from build123d import *

# Parameters (mm, degrees)
SKETCH_1_W          = 1150
SKETCH_1_H          = 15
EXTRUDE_1_DEPTH     = 30
SKETCH_2_R          = 7
CUT_EXTRUDE_1_DEPTH = 1195.521313651


with BuildPart() as part:
    # Эскиз1 → Бобышка-Вытянуть1 (new body)
    with BuildSketch(Plane.XY):
        with Locations((619.050320868, 30.131091658)):
            Rectangle(SKETCH_1_W, SKETCH_1_H)
    extrude(amount=EXTRUDE_1_DEPTH)

    # Эскиз2 → Вырез-Вытянуть1 (cut, through all)
    with BuildSketch(Plane(origin=(0, 37.631091658, 0), x_dir=(1, 0, 0), z_dir=(0, 1, 0))):
        with Locations(Location((144.050320868, -15, 0), (0, 0, 270))):
            Circle(SKETCH_2_R)
        with Locations(Location((614.050320868, -15, 0), (0, 0, 270))):
            Circle(SKETCH_2_R)
        with Locations(Location((1084.050320868, -15, 0), (0, 0, 270))):
            Circle(SKETCH_2_R)
    extrude(amount=-CUT_EXTRUDE_1_DEPTH, mode=Mode.SUBTRACT)


solid = part.part
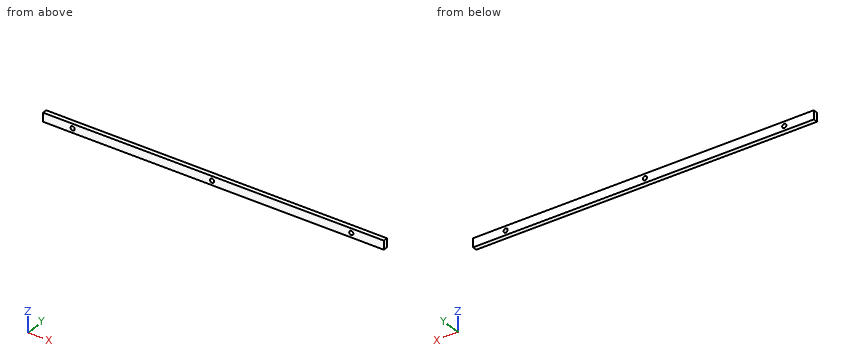
The model under review builds one solid part; all positions refer to its coordinate system, in mm. Give positions to 0.01 mm unless a question says otherwise; leave off trailing zeros. Order: outer loops, then holes, each group sorted by start corner. A loop starts at its lowest first (then second) coordinate and runs counter-clockwise, first axis right, second up. Notation, with made-up numbers: M 89.25,7.5 L 118.25,7.5 A18 cw 118.25,17.5 Z; hole C -30,50 d11. An arc over 180 degrees is marked long. Answer in a Markdown table with one row per item. Add a question column.
1. To check wall thickness, follow line 1 along X through (y, z) = (36, 15); line 2 along X through (y, z) = (35, 8.75). State the ranges of each line that lie inside material, in increasing order.
2. For pin 1 Ø11 at (x, z) = (1084.05, 15) entering from +Y, flat-tipped, find the tip position at first contact; note if it passes through.
3. Add section A-A on z = 15. State the section outline as (x, y) points, plus the area to 3 significant figures.
The answers:
| question | item | result |
|---|---|---|
| 1 | line 1 | 44.05 to 137.05, 151.05 to 607.05, 621.05 to 1077.05, 1091.05 to 1194.05 |
| 1 | line 2 | 44.05 to 140.9, 147.2 to 610.9, 617.2 to 1080.9, 1087.2 to 1194.05 |
| 2 | pin 1 | through |
| 3 | outline | M 44.05,22.63 L 137.05,22.63 L 137.05,37.63 L 44.05,37.63 Z; M 151.05,22.63 L 607.05,22.63 L 607.05,37.63 L 151.05,37.63 Z; M 621.05,22.63 L 1077.05,22.63 L 1077.05,37.63 L 621.05,37.63 Z; M 1091.05,22.63 L 1194.05,22.63 L 1194.05,37.63 L 1091.05,37.63 Z |
| 3 | area | 16,600 mm2 |
